Model file for the job. Use its own axes, mm. Give positions to 0.01 mm unless a question says otherwise; leave off trailing zeros. Order: outer loops, then holes, each group sorted by start corner. A loop starts at its lowest first (then second) coordinate and runs counter-clockwise, first axis right, second up. Notation, with made-up numbers: (-32.75, -11) -> (5.25, -11) arc R31 cw to (5.25, 25) -> close; hole circle Ø9 at (52, -14). An arc over 180 degrees is marked (long way). Answer in a Markdown table with one row per item. Add a question column.
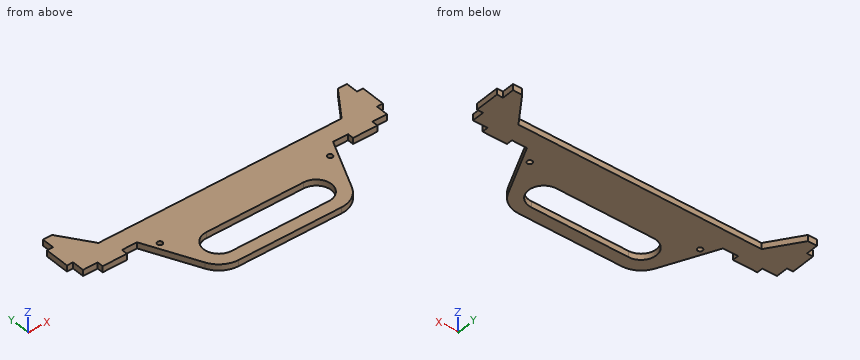
from build123d import *

# Parameters (mm, degrees)
BOSS_EXTRUDE1_DEPTH = 5
FILLET1_R           = 20
SKETCH3_R           = 2.1
CUT_EXTRUDE1_DEPTH  = 5


with BuildPart() as part:
    # Sketch1 → Boss-Extrude1 (new body)
    with BuildSketch(Plane.XY):
        Polygon((0, 0), (7.494811542, 0), (24.999999999, -25), (224.999999999, -25), (242.505188456, 0), (249.999999998, 0), (249.999999998, -10), (254.999999998, -10), (254.999999998, -30), (249.999999998, -30), (249.999999998, -40), (237.999999998, -40), (237.999999998, -45), (217.999999998, -45), (217.999999998, -40), (205.646921198, -40), (179.999999999, -95), (69.999999999, -95), (44.353078801, -40), (32, -40), (32, -45), (12, -45), (12, -40), (0, -40), (0, -30), (-5, -30), (-5, -10), (0, -10), align=None)
        with BuildLine():
            Line((84.999999999, -60), (164.999999999, -60))
            ThreePointArc((164.999999999, -60), (177.499999999, -72.5), (164.999999999, -85))
            Line((164.999999999, -85), (84.999999999, -85))
            ThreePointArc((84.999999999, -85), (72.499999999, -72.5), (84.999999999, -60))
        make_face(mode=Mode.SUBTRACT)
    extrude(amount=BOSS_EXTRUDE1_DEPTH)

    # Fillet1
    fillet1_edges = [part.edges().sort_by_distance(p)[0] for p in [
        (179.999999999, -95, 2.5),
        (69.999999999, -95, 2.5),
    ]]
    fillet(fillet1_edges, radius=FILLET1_R)

    # Sketch3 → Cut-Extrude1 (cut)
    with BuildSketch(Plane.XY.offset(5)):
        with Locations((55, -50)):
            Circle(SKETCH3_R)
    cut_extrude1 = extrude(amount=-CUT_EXTRUDE1_DEPTH, mode=Mode.SUBTRACT)

    # Mirror1: Cut-Extrude1 across plane
    add(cut_extrude1.mirror(Plane.ZY.offset(-124.999999999)), mode=Mode.SUBTRACT)


solid = part.part
Item 1: Pin check, flat tips, straight feed: pin 1 Ø2.5 at (x, z) = (-3.5, 2) entering from +Y; pin 2 Ø1.5 at (y, z) = (-43, 3) entering from -X; pin 3 Ø2.5 at (x, z) = (122, 3) entering from +Y; pin 4 Ø4 at (x, y) = (195, -50) entering from -Z. Stop position of each tip, or through.
Item 2: Saw through at B-B on y = -72.5. List the corners of the cut face in (x, z).
Item 3: Saw through at C-C on z = 3.65. Give the number of separate pieces and of enclosed holes in the cut face, plus the area to 3 significant figures.
Item 4: Saw through at A-A on x = 126. List the corners of the cut face in (y, z).
Item 5: Wall check: line 1 (Y direction, x = 119, z = 3.75); line 2 (X direction, y = -48.5, z = 1.35); line 3 (X direction, y = -49.5, z = 3.6). Give the ranges that are in metal, low to high.
Evaluation:
| question | item | result |
|---|---|---|
| 1 | pin 1 | stops at y = -10 |
| 1 | pin 2 | stops at x = 12 |
| 1 | pin 3 | stops at y = -25 |
| 1 | pin 4 | passes through |
| 2 | outline | (59.51, 0) -> (72.5, 0) -> (72.5, 5) -> (59.51, 5) -> close; (177.5, 0) -> (190.49, 0) -> (190.49, 5) -> (177.5, 5) -> close |
| 3 | separate pieces | 1 |
| 3 | enclosed holes | 3 |
| 3 | area | 9,850 mm2 |
| 4 | outline | (-95, 0) -> (-85, 0) -> (-85, 5) -> (-95, 5) -> close; (-60, 0) -> (-25, 0) -> (-25, 5) -> (-60, 5) -> close |
| 5 | line 1 | y = -95 to -85, -60 to -25 |
| 5 | line 2 | x = 48.32 to 53.53, 56.47 to 193.53, 196.47 to 201.68 |
| 5 | line 3 | x = 48.78 to 52.96, 57.04 to 192.96, 197.04 to 201.22 |
